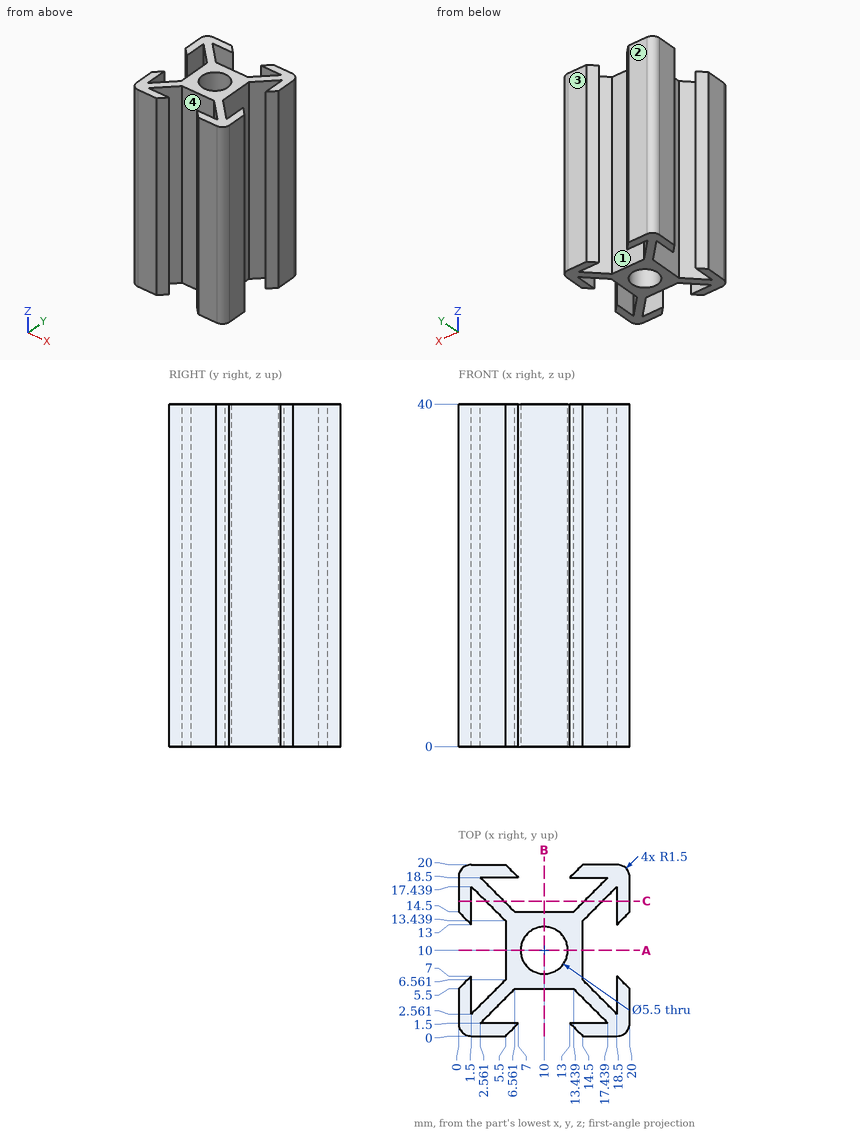
Design review of the part shown in the three views and the two pictorial views. Dimensions are in mm from the part's minimum x, y and z. A direction names the side the tool comes from. Round coordinates to 2 decimals unless told otherwise and drop trailing zeros. Write each loop counter-clockwise with the first axis right and the second up, starting at its lowest first coordinate (ties: lowest second). Pieces come first, ordered by that corner, then holes. Notation, with made-up numbers: (4.5, 15) - (58.5, 15) arc R20 cw to (58.5, 44) - close; hole circle Ø6 at (-8.75, 3). An arc over 180 degrees is marked (long way). Write item = value, one per line. Start each with the question number.
1. Consider section C-C on y = 15.75. State the section outline as (x, z) points.
2. Consider section A-A on y = 10. State the section outline as (x, z) points, plus the area to 3 significant figures.
3. Wall thickness on L1, parallel to Y at x = 10, z = 17.5; L2, parallel to Y at x = 14.75, z = 34.5; L3, parallel to Y at x = 16.25, z = 36: over which ranges is each line inside the solid? List them lowest first.
4. For pin 1 Ø1 at (x, z) = (8.5, 25.5) entering from +Y; pin 2 Ø2 at (y, z) = (8.5, 28) entering from -X; pin 3 Ø3.5 at (y, z) = (10, 23) entering from +X, all flat-tipped, find the tip position at first contact; note any pin that passes through.
5. For the marked faces 1 and 2, list the 3-axis set-ups (+Z, -Z, +X, -X, +Y, -Y) from which the entire face can be reached by the end or side of a thin tool; tool diameter is ignored.
6. Draft analysis for pull direction X (two halves, no side actions). For the marked faces 3 and 4, state which applies: released by +X, released by -X, zero draft, split by the parting line, or undercut.
Evaluation:
q1.outline = (0, 0) - (1.5, 0) - (1.5, 40) - (0, 40) - close; (3.19, 0) - (5.31, 0) - (5.31, 40) - (3.19, 40) - close; (14.69, 0) - (16.81, 0) - (16.81, 40) - (14.69, 40) - close; (18.5, 0) - (20, 0) - (20, 40) - (18.5, 40) - close
q2.outline = (5.5, 0) - (7.25, 0) - (7.25, 40) - (5.5, 40) - close; (12.75, 0) - (14.5, 0) - (14.5, 40) - (12.75, 40) - close
q2.area = 140 mm2
q3.L1 = 5.5 to 7.25, 12.75 to 14.5
q3.L2 = 0 to 1.5, 4.19 to 6.31, 13.69 to 15.81, 18.5 to 20
q3.L3 = 0 to 1.5, 2.69 to 4.81, 15.19 to 17.31, 18.5 to 20
q4.pin_1 = 14.5
q4.pin_2 = 5.5
q4.pin_3 = 14.5
q5.face_1 = +Z, -Z
q5.face_2 = +Z, -Z, +X, -X, +Y
q6.face_3 = zero draft
q6.face_4 = undercut
